from build123d import *

# Parameters (mm, degrees)
SKETCH1_W           = 6.5
SKETCH1_H           = 68.5
SKETCH1_W_2         = 3.5
SKETCH1_H_2         = 65.5
BOSS_EXTRUDE1_DEPTH = 6
SKETCH2_W           = 6.5
SKETCH2_H           = 68.5
BOSS_EXTRUDE2_DEPTH = 0.5
BOSS_EXTRUDE3_DEPTH = 1


with BuildPart() as part:
    # Sketch1 → Boss-Extrude1 (new body)
    with BuildSketch(Plane.XY):
        with Locations((3.25, 34.25)):
            Rectangle(SKETCH1_W, SKETCH1_H)
        with Locations((3.25, 34.25)):
            Rectangle(SKETCH1_W_2, SKETCH1_H_2, mode=Mode.SUBTRACT)
    extrude(amount=BOSS_EXTRUDE1_DEPTH)

    # Sketch2 → Boss-Extrude2 (add)
    with BuildSketch(Plane(origin=(0, 0, 0), x_dir=(-1, 0, 0), z_dir=(0, 0, -1))):
        with Locations((-3.25, 34.25)):
            Rectangle(SKETCH2_W, SKETCH2_H)
    extrude(amount=BOSS_EXTRUDE2_DEPTH)

    # Sketch3 → Boss-Extrude3 (add)
    with BuildSketch(Plane.ZY):
        with BuildLine():
            Line((1, 64), (1.5, 64))
            ThreePointArc((1.5, 64), (1.853553391, 63.853553391), (2, 63.5))
            Line((2, 63.5), (2, 63))
            ThreePointArc((2, 63), (1.853553391, 62.646446609), (1.5, 62.5))
            Line((1.5, 62.5), (1, 62.5))
            ThreePointArc((1, 62.5), (0.646446609, 62.646446609), (0.5, 63))
            Line((0.5, 63), (0.5, 63.5))
            ThreePointArc((0.5, 63.5), (0.646446609, 63.853553391), (1, 64))
        make_face()
        with BuildLine():
            Line((1, 6), (1.5, 6))
            ThreePointArc((1.5, 6), (1.853553391, 5.853553391), (2, 5.5))
            Line((2, 5.5), (2, 5))
            ThreePointArc((2, 5), (1.853553391, 4.646446609), (1.5, 4.5))
            Line((1.5, 4.5), (1, 4.5))
            ThreePointArc((1, 4.5), (0.646446609, 4.646446609), (0.5, 5))
            Line((0.5, 5), (0.5, 5.5))
            ThreePointArc((0.5, 5.5), (0.646446609, 5.853553391), (1, 6))
        make_face()
    extrude(amount=BOSS_EXTRUDE3_DEPTH)


solid = part.part
Part model, mm, in its own coordinate system. A direction names the side the tool comes from. Coordinates: 2 decimals unless noted, no trailing zeros. Loops run counter-clockwise (first coordinate to the right, second up) from the corner with the lowest first, then second, coordinate; pieces in that order, holes last. Notation, with made-up numbers: M 76.5,8.5 L 126.5,8.5 A37 cw 126.5,46.5 Z; hole C 66,7 d5. An arc over 180 degrees is marked long. Use a Markdown table: item, result. Add a question column.
Q1. Pin check, flat tips, straight feed: P1, Ø0.6, axis at x = -0.5, y = 5.5, coming from the -Z side; P2, Ø1, axis at x = 4, y = 29.5, coming from the +Z side. Stop position of each tip, or through.
Q2. Mould opens along Y. For faces 1 (the flat face through (3, 1.5, 3)), 2 (the flat face through (3, 68.5, 3)), 3 (the flat face through (3, 0, 3)) say: +Y half, -Y half, draft (parallel to the pull), parting line (faces both ways), or undercut.
Q3. Probe L1, parallel to Y at x = 2.25, z = 1; L2, parallel to X at y = 60, z = 5.75; L3, parallel to Y at x = -0.5, z = 1. List the from-to ranges inside material, lowest first.
Q4. Cut at A-A (z = 5). Write the cut outline in (x, y), and give its area (3 significant figures).
Q5. Cut at B-B (y = 23.5). Write the cut outline in (x, z).
Q6. Cut at C-C (x = 4). Write the cut outline in (y, z).
Q7. Which spindle directions (+Z, -Z, +X, -X, +Y, -Y) get a long thin tool onto all of the face, cutting with end or side? Do faces 4 (the flat face through (-1, 5, 1)), 5 (the flat face through (3, 35, 0)). Say none if no direction does.
Worked out:
| question | item | result |
|---|---|---|
| 1 | P1 | stops at z = 0.5 |
| 1 | P2 | stops at z = 0 |
| 2 | face 1 | undercut |
| 2 | face 2 | +Y half |
| 2 | face 3 | -Y half |
| 3 | L1 | y = 0 to 1.5, 67 to 68.5 |
| 3 | L2 | x = 0 to 1.5, 5 to 6.5 |
| 3 | L3 | y = 4.5 to 6, 62.5 to 64 |
| 4 | outline | M 0,0 L 6.5,0 L 6.5,68.5 L 0,68.5 Z; hole M 1.5,1.5 L 5,1.5 L 5,67 L 1.5,67 Z |
| 4 | area | 216 mm2 |
| 5 | outline | M 0,-0.5 L 6.5,-0.5 L 6.5,6 L 5,6 L 5,0 L 1.5,0 L 1.5,6 L 0,6 Z |
| 6 | outline | M 0,-0.5 L 68.5,-0.5 L 68.5,6 L 67,6 L 67,0 L 1.5,0 L 1.5,6 L 0,6 Z |
| 7 | face 4 | +Z, -Z, -X, +Y, -Y |
| 7 | face 5 | +Z |
